The model under review builds one solid part; all positions refer to its coordinate system, in mm. Face numbers are marked on the shaded views. Coordinates: 2 decimals unless noted, no trailing zeros. Loops run counter-clockwise (first coordinate to the right, second up) from the corner with the lowest first, then second, coordinate; pieces in that order, holes last. Notation, with made-up numbers: (15.25, -36) - (25.25, -36) arc R11 cw to (25.25, -17) - close; hole circle Ø1 at (-11, -1.75). An arc over 180 degrees is marked (long way). One line per item, written item: value. Start each with the question number.
1. To check wall thickness, follow line 1 (Z direction, x = 16, y = 3.5); line 2 (Z direction, x = 1, y = 2.25); line 3 (X direction, y = 5.15, z = 0). State the ranges of each line that lie inside material, in increasing order.
2. Mouldability with a two-part tool opening along Y and no side actions: class the marked faces 1, 2 and 3 as +Y half, -Y half, draft (parallel to the pull), parting line (faces both ways), or undercut.
3. We need section C-C, the plane y = 4. Give the boundary of the cut face in (x, z).
4. We need section D-D, the plane z = -16. Give the boundary of the cut face in (x, y).
5. Insertion check: P1, Ø4, axis at y = 5.5, z = 9, coming from the -X side (3 decimals); P2, Ø12, axis at x = 12, z = 5, coming from the +Y side; P3, Ø0.8, axis at x = 13.5, y = 1, coming from the +Z side. Each pin has a flat end and moves straight along its axis. Give the tip position at first contact, or say it passes through.
6. We need section A-A, the plane y = 6.5. Give the boundary of the cut face in (x, z), then the cut area to 3 significant figures.
7. We need section B-B, the plane z = -1. Give the boundary of the cut face in (x, y).
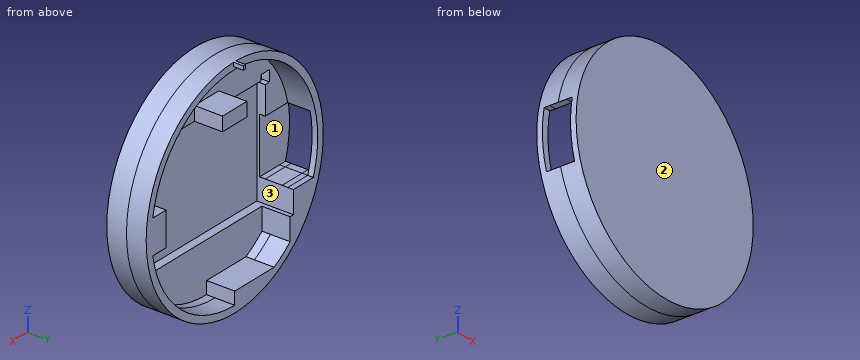
Autodesk Inventor part; units mm, degrees
ref_plane "Work Plane1" through (0, 3.5, 0) normal (0, 1, 0) x (1, 0, 0)
ref_plane "YZ Plane" through (0, 0, 0) normal (1, 0, 0) x (0, 1, 0)
ref_plane "XZ Plane" through (0, 0, 0) normal (0, 1, 0) x (-1, 0, 0)
sketch "Sketch1" plane through (0, 0, 0) normal (0, 1, 0) x (-1, 0, 0)
  circle A0 centre (0, 0) radius 20
  dimension "d0" = 40
extrude "Extrusion1" add sketch "Sketch1" along normal blind 0.5
sketch "Sketch2" plane through (0, 0.5, 0) normal (0, 1, 0) x (1, 0, 0)
  line L0 (-13.25, -10) -> (13.25, -10)
  line L1 (13.25, -10) -> (13.25, 10)
  line L2 (13.25, 10) -> (-13.25, 10)
  line L3 (-13.25, 10) -> (-13.25, -10)
  line L4 (-13.25, -10) -> (13.25, 10) construction
  line L5 (13.25, -10) -> (-13.25, 10) construction
  circle A0 centre (0, 0) radius 20
  dimension "d3" = 26.5
  dimension "d4" = 20
extrude "Extrusion2" add sketch "Sketch2" along normal blind 3
ref_plane "Work Plane1" through (0, 3.5, 0) normal (0, 1, 0) x (1, 0, 0)
sketch "Sketch3" plane through (0, 3.5, 0) normal (0, 1, 0) x (1, 0, 0)
  line L0 (16.25, 0) -> (16.25, 3)
  line L1 (16.25, 3) -> (18.2551, 3)
  line L2 (16.25, 0) -> (16.25, -3)
  line L3 (16.25, -3) -> (18.2551, -3)
  line L4 (0, -18.5) -> (0, -12.5)
  line L5 (0, -12.5) -> (2.75, -12.5)
  line L6 (2.75, -12.5) -> (-2.75, -12.5)
  line L7 (-2.75, -12.5) -> (-2.75, -10)
  line L8 (-2.75, -10) -> (2.75, -10)
  line L9 (2.75, -10) -> (2.75, -12.5)
  line L10 (-17.5, 6) -> (-13.25, 6)
  line L11 (-12.5, 10) -> (-12.5, 13.6382)
  line L12 (0, 18.5) -> (0, 16.5)
  line L13 (0, 16.5) -> (-8.3666, 16.5)
  line L14 (18.2551, -3) -> (15.4901, -3)
  line L15 (15.4901, -3) -> (15.4901, 3)
  line L16 (15.4901, 3) -> (16.25, 3)
  circle A0 centre (0, 0) radius 18.75
  line L17 (18.2551, 3) -> (18.5084, 3)
  line L18 (18.2551, -3) -> (18.5084, -3)
  line L19 (0, 18.5) -> (0, 18.75)
  line L20 (-8.3666, 16.5) -> (-8.9058, 16.5)
  line L21 (-17.5, 6) -> (-17.7641, 6)
  line L22 (-12.5, 13.6382) -> (-12.5, 13.9754)
  line L23 (-13.25, 10) -> (13.25, 10)
  line L24 (-12.5, 10) -> (-13.25, 10)
  line L25 (-13.25, 10) -> (-13.25, 6)
  line L26 (-13.25, -10) -> (-13.25, 10)
  circle A1 centre (0, 0) radius 20
  dimension "d8" = 6
  dimension "d9" = 2.75
  dimension "d10" = 5.5
  dimension "d11" = 2
  dimension "d12" = 2.765
  dimension "d13" = 37.5
extrude "Extrusion3" cut sketch "Sketch3" against normal blind 1.5 contours L16 L15 L14 L3 L18 A0 L21 L10 L25 L23 L11 L22 L20 L13 L12 L19 L17 L1
extrude "Extrusion4" add sketch "Sketch3" along normal blind 5.25 contours L2 L14 L15 L16 L0 | L0 L1 L17 A0 L18 L3 L2 | L19 L12 L13 L20 A0 | A0 L22 L11 L23 L25 L10 L21 | L6 L7 L8 L9 L5
extrude "Extrusion5" add sketch "Sketch3" along normal blind 5.25 contours A1
sketch "Sketch4" plane through (0, 2, 0) normal (0, 1, 0) x (1, 0, 0)
  line L0 (14.25, -9) -> (12.25, -9)
  line L1 (12.25, -9) -> (12.25, -11)
  line L2 (12.25, -11) -> (14.25, -11)
  line L3 (14.25, -11) -> (14.25, -9)
  line L4 (2.75, -10) -> (13.25, -10)
  line L5 (14.25, -9) -> (12.25, -11) construction
  line L6 (12.25, -9) -> (14.25, -11) construction
  point P0 (0, 0)
  dimension "d20" = 2
  dimension "d21" = 2
extrude "Extrusion6" cut sketch "Sketch4" against normal blind 1.5
sketch "Sketch5" plane through (0, 8.75, 0) normal (0, 1, 0) x (1, 0, 0)
  circle A0 centre (0, 0) radius 19.25
  circle A1 centre (0, 0) radius 20
  circle A2 centre (0, 0) radius 19.5
  dimension "d24" = 38.5
  dimension "d25" = 39
extrude "Extrusion7" add sketch "Sketch5" along normal blind 5 contours A1 | A2
extrude "Extrusion8" add sketch "Sketch5" along normal blind 6 contours A1
sketch "Sketch6" plane through (0, 14.75, 0) normal (0, 1, 0) x (1, 0, 0)
  line L0 (-0.2579, -20.6923) -> (0.2579, -20.6923)
  line L1 (0.2579, -20.6923) -> (0.2579, -19.3077)
  line L2 (0.2579, -19.3077) -> (-0.2579, -19.3077)
  line L3 (-0.2579, -19.3077) -> (-0.2579, -20.6923)
  circle A0 centre (0, 0) radius 20
  line L4 (-0.2579, -20.6923) -> (0.2579, -19.3077) construction
  line L5 (0.2579, -20.6923) -> (-0.2579, -19.3077) construction
  point P0 (0, -20)
  point P1 (0.2579, -19.9983)
  point P2 (-0.2579, -19.9983)
extrude "Extrusion9" add sketch "Sketch6" along normal blind 1 contours L3 A0 L1 L0 | L3 L2 L1 A0 picked at (-0.0287, -19.5384)
sketch "Sketch7" plane through (0.2579, 14.75, 20.6923) normal (1, 0, 0) x (0, 0, -1)
  line L0 (0, 0) -> (0.6939, 0)
  line L1 (0.6939, 0) -> (0.9439, 0)
  line L2 (1.194, 0) -> (0.6939, 0)
  circle A0 centre (0.9439, 0) radius 0.25
  line L3 (1.194, 0) -> (1.3845, 0)
  line L4 (1.194, 0) -> (2.041, 0)
  point P0 (20.6923, -14.75)
  point P1 (0.6939, 0)
  dimension "d32" = 0.25
extrude "Extrusion10" cut sketch "Sketch6" along normal blind 1 contours L3 A0 L1 L0 | L3 L2 L1 A0 picked at (-0.0287, -19.5384)
sketch "Sketch8" plane through (0, 2, 0) normal (0, 1, 0) x (1, 0, 0)
  line L0 (-17.7641, 6) -> (-13.25, 6)
  line L1 (-13.25, 6) -> (-22.0504, 6)
  line L2 (-22.0504, 6) -> (-22.0504, -4)
  line L3 (-22.0504, -4) -> (-13.25, -4)
  line L4 (-13.25, -4) -> (-13.25, 6)
  point P0 (0, 0)
  dimension "d37" = 10
extrude "Extrusion11" cut sketch "Sketch8" against normal blind 1
extrude "Extrusion12" cut sketch "Sketch8" along normal blind 3
extrude "Extrusion13" cut sketch "Sketch8" along normal blind 4
sketch "Sketch9" plane through (0, 2, 0) normal (0, 1, 0) x (1, 0, 0)
  line L0 (-12.25, -11) -> (-14.25, -11)
  line L1 (-14.25, -11) -> (-14.25, -9)
  line L2 (-14.25, -9) -> (-12.25, -9)
  line L3 (-12.25, -9) -> (-12.25, -11)
  line L4 (-12.25, -11) -> (-14.25, -9) construction
  line L5 (-14.25, -11) -> (-12.25, -9) construction
  point P0 (0, 0)
  point P1 (-13.25, -10)
  dimension "d44" = 2
  dimension "d45" = 2
extrude "Extrusion14" cut sketch "Sketch9" against normal blind 1.5
extrude "Extrusion15" cut sketch "Sketch6" against normal blind 7.75 contours A0 L1 L2 L3 picked at (-0.5744, 6.7866)
extrude "Extrusion16" cut sketch "Sketch5" along normal blind 7.75 contours A0 | A1 | A2
properties part number "t2"
Findings below:
1. line 1: -12 to -9.78, -3 to 3, 9.78 to 12
1. line 2: -19.97 to -18.72, 10 to 12.5, 18.72 to 19.97
1. line 3: 15.49 to 20
2. face 1: undercut
2. face 2: -Y half
2. face 3: draft
3. outline: (-19.6, 4) - (-18.32, 4) arc R18.75 cw to (18.51, 3) - (15.49, 3) - (15.49, -3) - (18.51, -3) arc R18.75 cw to (0, -18.75) - (0, -16.5) - (-8.91, -16.5) arc R18.75 cw to (-12.5, -13.98) - (-12.5, -10) - (-13.25, -10) - (-13.25, -6) - (-19.08, -6) arc R20 ccw (long way) to start; (-2.75, 10) - (2.75, 10) - (2.75, 12.5) - (-2.75, 12.5) - close
4. outline: (-12, 0) - (12, 0) - (12, 7) - (9.78, 7) - (9.78, 2) - (-9.78, 2) - (-9.78, 7) - (-12, 7) - close
5. P1: x = -18.735
5. P2: y = 7
5. P3: z = 15.11
6. outline: circle Ø40 at (0, 0); (-2.75, 10) - (2.75, 10) - (2.75, 12.5) - (-2.75, 12.5) - close; hole (-17.76, -6) - (-13.25, -6) - (-13.25, -10) - (-12.5, -10) - (-12.5, -13.98) arc R18.75 ccw to (-8.91, -16.5) - (0, -16.5) - (0, -18.75) arc R18.75 ccw to (18.51, -3) - (15.49, -3) - (15.49, 3) - (18.51, 3) arc R18.75 ccw (long way) to start
6. area: 220 mm2
7. outline: (-19.97, 0) - (19.97, 0) - (19.97, 7) - (15.49, 7) - (15.49, 2) - (13.25, 2) - (13.25, 0.5) - (-13.25, 0.5) - (-13.25, 1) - (-19.97, 1) - close; (-19.97, 6) - (-18.72, 6) - (-18.72, 7) - (-19.97, 7) - close
